Verification items for this drawing (mm, ordinates from the low corner). Round coordinates to 2 decimals unless told otherwise and drop trailing zeros. Loops run counter-clockwise (first coordinate to the right, second up) from the corner with the lowest first, then second, coordinate; pieces in that order, holes last. Notation, with made-up numbers: (-24.5, -14.5) - (-6.5, -14.5) arc R25 cw to (-6.5, 20.5) - close; hole circle Ø9 at (24.5, 5.25). An arc over 180 degrees is marked (long way). Use a Markdown table: item, result. Add a question column.
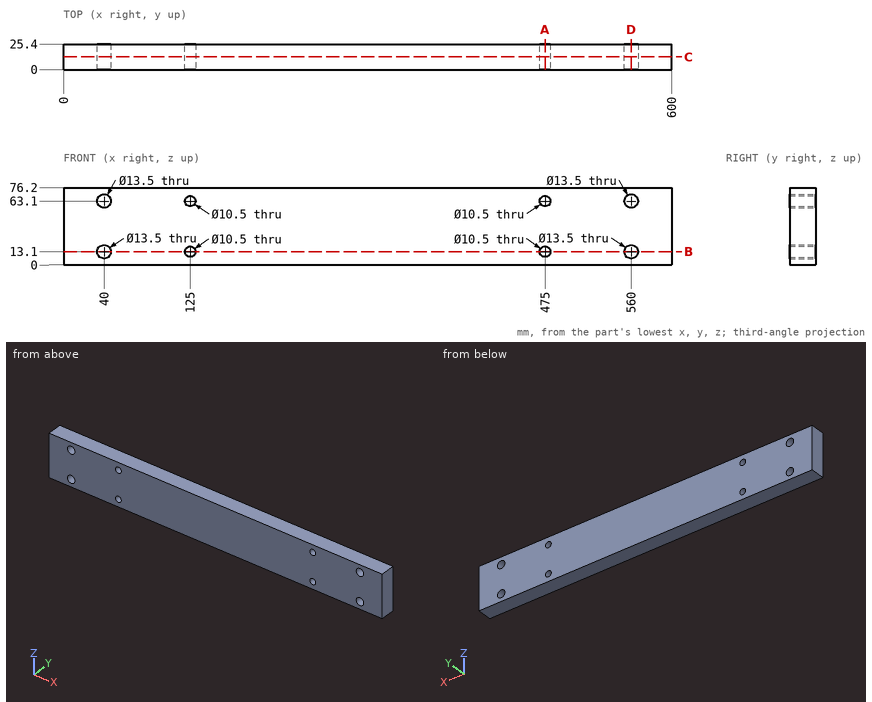
Q1. Section check C-C on y = 12.75. State how many separate pieces and enclosed holes the cut face has, plus the area to 3 significant figures.
Q2. Section check D-D on x = 560. Record the cut outline in (y, z).
Q3. Section check B-B on z = 13.1. Record the cut outline in (x, y), plus the area to 3 significant figures.
Q4. Thickness scan on line 1 along Z through (x, y) = (475, 13.75); line 2 along X through (y, z) = (2, 14); line 3 along Z through (x, y) = (560, 17.5). Record the ranges inside material, lowest first.
Q5. Section check A-A on x = 475. Record the cut outline in (y, z), plus the area to 3 significant figures.
Determined:
| question | item | result |
|---|---|---|
| 1 | separate pieces | 1 |
| 1 | enclosed holes | 8 |
| 1 | area | 44,800 mm² |
| 2 | outline | (0, 0) - (25.4, 0) - (25.4, 6.35) - (0, 6.35) - close; (0, 19.85) - (25.4, 19.85) - (25.4, 56.35) - (0, 56.35) - close; (0, 69.85) - (25.4, 69.85) - (25.4, 76.2) - (0, 76.2) - close |
| 3 | outline | (0, 0) - (33.25, 0) - (33.25, 25.4) - (0, 25.4) - close; (46.75, 0) - (119.75, 0) - (119.75, 25.4) - (46.75, 25.4) - close; (130.25, 0) - (469.75, 0) - (469.75, 25.4) - (130.25, 25.4) - close; (480.25, 0) - (553.25, 0) - (553.25, 25.4) - (480.25, 25.4) - close; (566.75, 0) - (600, 0) - (600, 25.4) - (566.75, 25.4) - close |
| 3 | area | 14,000 mm² |
| 4 | line 1 | z = 0 to 7.85, 18.35 to 57.85, 68.35 to 76.2 |
| 4 | line 2 | x = 0 to 33.31, 46.69 to 119.83, 130.17 to 469.83, 480.17 to 553.31, 566.69 to 600 |
| 4 | line 3 | z = 0 to 6.35, 19.85 to 56.35, 69.85 to 76.2 |
| 5 | outline | (0, 0) - (25.4, 0) - (25.4, 7.85) - (0, 7.85) - close; (0, 18.35) - (25.4, 18.35) - (25.4, 57.85) - (0, 57.85) - close; (0, 68.35) - (25.4, 68.35) - (25.4, 76.2) - (0, 76.2) - close |
| 5 | area | 1,400 mm² |
